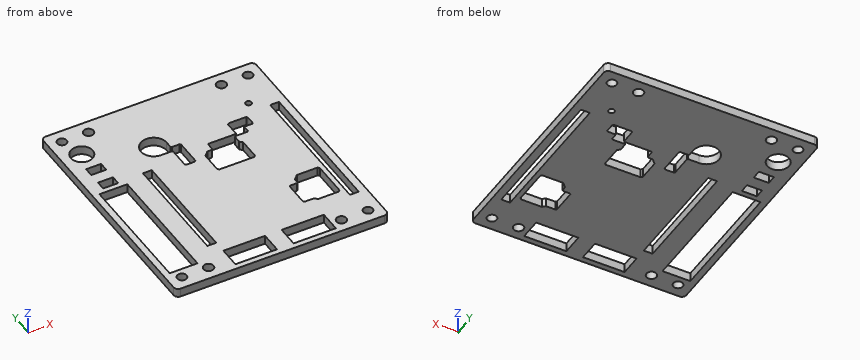
from build123d import *

# Parameters (mm, degrees)
MODEL_R                 = 1
MODEL_R_2               = 3.7
MODEL_R_3               = 1.7
MODEL_R_4               = 1.600279216
MODEL_W                 = 3
MODEL_H                 = 47.88
MODEL_H_2               = 38.677610829
MODEL_W_2               = 14.305297
MODEL_H_3               = 7.199932059
MODEL_W_3               = 14.105297
MODEL_W_4               = 5.1
MODEL_H_4               = 3.1
SALIENTE_EXTRUIR1_DEPTH = 3


with BuildPart() as part:
    # Model → Saliente-Extruir1 (new body)
    with BuildSketch(Plane.XY):
        with BuildLine():
            Line((79.069803803, 220.603820632), (79.069803803, 298.60843049))
            ThreePointArc((79.069803803, 298.60843049), (78.630463975, 299.669090662), (77.569803803, 300.10843049))
            Line((77.569803803, 300.10843049), (8.567399569, 300.10843049))
            ThreePointArc((8.567399569, 300.10843049), (7.506739397, 299.669090662), (7.067399569, 298.60843049))
            Line((7.067399569, 298.60843049), (7.067399569, 220.603820632))
            ThreePointArc((7.067399569, 220.603820632), (7.506739397, 219.54316046), (8.567399569, 219.103820632))
            Line((8.567399569, 219.103820632), (77.569803803, 219.103820632))
            ThreePointArc((77.569803803, 219.103820632), (78.630463975, 219.54316046), (79.069803803, 220.603820632))
        make_face()
        with Locations((68.304134727, 284.23112787)):
            Circle(MODEL_R, mode=Mode.SUBTRACT)
        with Locations((13.830317101, 287.723880192)):
            Circle(MODEL_R_2, mode=Mode.SUBTRACT)
        with Locations((20.566730565, 223.60348613)):
            Circle(MODEL_R_3, mode=Mode.SUBTRACT)
        with Locations((65.570138305, 223.60348613)):
            Circle(MODEL_R_3, mode=Mode.SUBTRACT)
        with Locations((11.567065067, 223.60348613)):
            Circle(MODEL_R_4, mode=Mode.SUBTRACT)
        with Locations((74.569803803, 223.60348613)):
            Circle(MODEL_R_4, mode=Mode.SUBTRACT)
        with Locations((20.566730565, 295.60843049)):
            Circle(MODEL_R_3, mode=Mode.SUBTRACT)
        with Locations((65.570138305, 295.60843049)):
            Circle(MODEL_R_3, mode=Mode.SUBTRACT)
        with Locations((74.569803803, 295.60843049)):
            Circle(MODEL_R_4, mode=Mode.SUBTRACT)
        with Locations((11.567065067, 295.60843049)):
            Circle(MODEL_R_4, mode=Mode.SUBTRACT)
        with Locations((74.943202287, 256.416250186)):
            Rectangle(MODEL_W, MODEL_H, mode=Mode.SUBTRACT)
        with Locations((26.680813222, 251.818953656)):
            Rectangle(MODEL_W, MODEL_H_2, mode=Mode.SUBTRACT)
        Polygon((9.255063306, 269.010369093), (9.256333369, 226.883193232), (18.686310635, 226.883193232), (18.685040572, 269.010369093), align=None, mode=Mode.SUBTRACT)
        with BuildLine():
            Line((37.928978937, 268.658416829), (37.930092901, 275.569446794))
            Line((37.930092901, 275.569446794), (37.630141257, 275.86944679))
            Line((37.630141257, 275.86944679), (33.962054567, 275.86944679))
            ThreePointArc((33.962054567, 275.86944679), (30.886140069, 283.295361288), (38.312054567, 280.21944679))
            Line((38.312054567, 280.21944679), (38.312054567, 277.90087731))
            Line((38.312054567, 277.90087731), (38.612054567, 277.60087731))
            Line((38.612054567, 277.60087731), (41.272484784, 277.60087731))
            Line((41.272484784, 277.60087731), (41.572484784, 277.30087731))
            Line((41.572484784, 277.30087731), (41.572484784, 268.658416833))
            Line((41.572484784, 268.658416833), (41.272484784, 268.358416833))
            Line((41.272484784, 268.358416833), (38.228930581, 268.358416833))
            Line((38.228930581, 268.358416833), (37.928978937, 268.658416829))
        make_face(mode=Mode.SUBTRACT)
        with Locations((55.052147548, 224.605565735)):
            Rectangle(MODEL_W_2, MODEL_H_3, mode=Mode.SUBTRACT)
        with Locations((35.246780171, 224.605565735)):
            Rectangle(MODEL_W_3, MODEL_H_3, mode=Mode.SUBTRACT)
        with Locations((14.057658355, 272.349769149)):
            Rectangle(MODEL_W_4, MODEL_H_4, mode=Mode.SUBTRACT)
        with Locations((14.057658355, 279.495142856)):
            Rectangle(MODEL_W_4, MODEL_H_4, mode=Mode.SUBTRACT)
        Polygon((45.217053505, 262.162824271), (45.717053505, 261.662824271), (57.517053505, 261.662824271), (58.017053505, 262.162824271), (58.017053505, 269.162824271), (57.139240746, 270.040637031), (57.139240746, 272.521816974), (57.439240746, 272.821816974), (61.516534187, 272.821816974), (61.816534188, 273.121816974), (61.816534188, 275.340900661), (64.597764426, 275.340900661), (64.897764426, 275.640900661), (64.897764426, 278.38346156), (64.685649489, 278.89561069), (64.596997018, 278.984277451), (58.773973289, 278.984277451), (58.261824159, 278.772162514), (58.173924933, 278.684277455), (58.173157398, 273.922486249), (57.873109042, 273.622486253), (48.826048419, 273.622486253), (48.526048419, 273.322486253), (48.526048419, 270.962824271), (48.226048419, 270.662824271), (46.717053505, 270.662824271), (45.217053505, 269.162824271), align=None, mode=Mode.SUBTRACT)
        Polygon((63.45410467, 236.265050938), (60.172255448, 236.265050938), (59.872255448, 236.565050938), (59.872255448, 244.578243265), (60.172255448, 244.878243265), (62.53191743, 244.878243265), (62.83191743, 245.178243265), (62.83191743, 246.687238178), (64.33191743, 248.187238178), (71.33191743, 248.187238178), (71.83191743, 247.687238178), (71.83191743, 235.887238179), (71.33191743, 235.387238179), (64.33191743, 235.387238179), align=None, mode=Mode.SUBTRACT)
    extrude(amount=SALIENTE_EXTRUIR1_DEPTH)


solid = part.part
Input: part model. Units: mm. Frame: model coordinates. Coordinates: 2 decimals unless noted, no trailing zeros. Loops run counter-clockwise (first coordinate to the right, second up) from the corner with the lowest first, then second, coordinate; pieces in that order, holes last. Notation, with made-up numbers: (79, -3.5) -> (91, -3.5) arc R20 cw to (91, 11.5) -> close; hole circle Ø11 at (5.25, -15). An arc over 180 degrees is marked (long way). Write each question's results on one line, items separated by ' | '. Start each with the question number.
Q1. Section A-A, the plane y = 257. Return the cut outline in (x, z).
Q2. Ray query, line 1 (X direction, y = 228, z = 1.95); line 2 (X direction, y = 235, z = 0.95); line 3 (X direction, y = 263, z = 0.55). Return the intervals inside material, ascending. Write a range as from..to.
Q3. Section B-B, the plane z = 0.5. State how many separate pieces and enclosed holes the cut face has, plus the area to 3 significant figures.
Found:
1) outline: (7.07, 0) -> (9.26, 0) -> (9.26, 3) -> (7.07, 3) -> close; (18.69, 0) -> (25.18, 0) -> (25.18, 3) -> (18.69, 3) -> close; (28.18, 0) -> (73.44, 0) -> (73.44, 3) -> (28.18, 3) -> close; (76.44, 0) -> (79.07, 0) -> (79.07, 3) -> (76.44, 3) -> close
2) line 1: 7.07..9.26, 18.69..28.19, 42.3..47.9, 62.2..79.07 | line 2: 7.07..9.26, 18.69..25.18, 28.18..73.44, 76.44..79.07 | line 3: 7.07..9.26, 18.69..25.18, 28.18..45.22, 58.02..73.44, 76.44..79.07
3) separate pieces: 1 | enclosed holes: 20 | area: 4,420 mm2
